Autodesk Fusion 360 part; units mm, degrees
sketch "Sketch1" plane through (0, 0, 0) normal (0, 1, 0) x (1, 0, 0)
  circle A0 centre (0, 0) radius 48
  circle A1 centre (0, 0) radius 53
  dimension "d1" = 96
  dimension "d2" = 106
extrude "Extrude4" add sketch "Sketch1" along normal blind 10
sketch "Sketch4" plane through (0, 10, 0) normal (0, 1, 0) x (-1, 0, 0)
  circle A0 centre (0, 0) radius 48
  circle A1 centre (0, 0) radius 53
  line L0 (48, 0) -> (41.779, 0)
  line L1 (48, 0) -> (32.779, 0)
  circle A2 centre (40.279, 0) radius 1.5
  line L2 (-48, 0) -> (-32.779, 0)
  line L3 (-48, 0) -> (-41.779, 0)
  circle A3 centre (-40.279, 0) radius 1.5
  line L4 (32.779, 35.0648) -> (49, 35.0648)
  line L5 (49, 35.0648) -> (49, -35)
  line L6 (49, -35) -> (32.779, -35)
  line L7 (32.779, -35) -> (32.779, 35.0648)
  line L8 (-32.779, 35.0648) -> (-52, 35.0648)
  line L9 (-52, 35.0648) -> (-52, -35)
  line L10 (-52, -35) -> (-32.779, -35)
  line L11 (-32.779, -35) -> (-32.779, 35.0648)
  dimension "d13" = 6.221
  dimension "d14" = 15.221
  dimension "d15" = 3
  dimension "d16" = 15.221
  dimension "d17" = 6.221
  dimension "d18" = 3
extrude "Extrude5" add sketch "Sketch4" along normal blind 5 contours A0 L0 L1 A2 L7 | A0 A1 L4 L5 L6 | A0 L0 L1 A2 L6 L7 | A0 A1 L4 L8 | A0 A1 L6 L10 | A0 L2 L3 A3 L11 | A0 A1 L8 L9 L10 | A0 L2 L3 A3 L10 L11 | A1 L5 | A1 L9
sketch "Sketch5" plane through (0, 15, 0) normal (0, 1, 0) x (-1, 0, 0)
  circle A0 centre (40.279, 0) radius 1.5
  arc A1 (-32.8481, -35) -> (32.8481, -35) centre (0, 0) ccw
  line L0 (-32.8481, -35) -> (-32.779, -35)
  line L1 (-32.779, -35) -> (-32.779, 35.0648)
  arc A2 (32.779, 35.0648) -> (-32.779, 35.0648) centre (0, 0) ccw
  line L2 (32.779, 35.0648) -> (32.779, -35)
  line L3 (32.779, -35) -> (32.8481, -35)
  circle A3 centre (-40.279, 0) radius 1.5
  circle A4 centre (0, 0) radius 53
  circle A5 centre (0, 0) radius 48
extrude "Extrude6" add sketch "Sketch5" along normal blind 30 contours A4
thread "Thread1" thread offset 0 thread length 10
Part model, mm, in its own coordinate system. A direction names the side the tool comes from. Round coordinates to 2 decimals unless told otherwise and drop trailing zeros. Write each loop counter-clockwise with the first axis right and the second up, starting at its lowest first coordinate (ties: lowest second). Pieces come first, ordered by that corner, then holes. Notation, with made-up numbers: M 70,38 L 96,38 A20 ccw 96,75 Z; hole C 25,84 d4. An arc over 180 degrees is marked long. Return JSON: item names as keys, results as strings. Group by question number.
(1) Drill centre lines: probe 1 along X at (y, z) = (13.3, 0); probe 2 along Z at (x, y) = (0.5, 6.5). Where is each one in solid material? Low to high.
(2) Pin check, flat tips, straight feed: pin 1 Ø12 at (x, y) = (-3, 20.5) entering from -Z; pin 2 Ø4.5 at (x, z) = (-38.5, -1.5) entering from -Y; pin 3 Ø2.5 at (y, z) = (13, 17) entering from +X; pin 4 Ø16.5 at (x, z) = (-40, 9.5) entering from +Y. Stop position of each tip, or through.
(3) Saw through at B-B on y = 32. Write the cut outline in (x, z).
(4) Saw through at D-D on z = 12. Write the cut outline in (x, y).
(5) Saw through at A-A on z = 38. Write the cut outline in (x, y), then the cut area to 3 significant figures.
(6) Two-plate mould, pull along X, no slides. Class faces 5 (the face through (-28, 0, -40)), 6 (the face through (-0.506, 29.79, -47.997)): +X half, -X half, draft (parallel to the pull), parting line (faces both ways), or undercut.
(7) Which spindle directions (+Z, -Z, +X, -X, +Y, -Y) get a long thin tool onto all of the face, cutting with end or side? Do faces 1 (the face through (28, 45, 40)), 2 (the face through (-38.6, 10, 0.5)), 3 (the face through (47.997, 29.79, -0.502)), 4 (the face through (-32.779, 12, 0)). Say none if no direction does.
Returned:
{
 "1": {"probe 1": "-53 to -41.78, -38.78 to -32.78, 32.78 to 38.78, 41.78 to 53", "probe 2": "-53 to -48, 48 to 53"},
 "2": {"pin 1": "z = -53", "pin 2": "y = 10", "pin 3": "x = 50.61", "pin 4": "y = 45"},
 "3": {"outline": "C 0,0 d106; hole M -32.85,-35 A48 ccw 32.85,-35 A48 ccw 32.78,35.06 A48 ccw -32.78,35.06 A48 ccw Z"},
 "4": {"outline": "M -51.62,0 L -46.48,0 L -46.48,10 L -32.78,10 L -32.78,15 L -46.48,15 L -46.48,45 L -51.62,45 Z; M 32.78,10 L 46.48,10 L 46.48,0 L 51.62,0 L 51.62,45 L 46.48,45 L 46.48,15 L 32.78,15 Z"},
 "5": {"outline": "M -36.95,0 L -29.33,0 L -29.33,45 L -36.95,45 Z; M 29.33,0 L 36.95,0 L 36.95,45 L 29.33,45 Z", "area": "686 mm²"},
 "6": {"face 5": "draft", "face 6": "undercut"},
 "7": {"face 1": "+Z, -Z, +X, -X, +Y", "face 2": "-Y", "face 3": "+Y", "face 4": "+Y, -Y"}
}
